Verification items for the finished model (mm, model axes). A direction names the side the tool comes from. Round coordinates to 2 decimals unless told otherwise and drop trailing zeros. Write each loop counter-clockwise with the first axis right and the second up, starting at its lowest first coordinate (ties: lowest second). Pieces come first, ordered by that corner, then holes. Notation, with made-up numbers: (52, -5.75) - (100, -5.75) arc R16 cw to (100, 19.25) - close; hole circle Ø7 at (89.25, 61.5). An arc over 180 degrees is marked (long way). Answer as a JSON object with one key per item and string values.
```python
from build123d import *

# Parameters (mm, degrees)
SKETCH_1_R          = 12.25
SKETCH_1_R_2        = 1.25
EXTRUDE_1_DEPTH     = 2
SKETCH_2_R          = 3
EXTRUDE_2_DEPTH     = 10.63
SKETCH_3_W          = 2
SKETCH_3_H          = 12
EXTRUDE_3_DEPTH     = 8
SKETCH_5_R          = 1.6
CUT_EXTRUDE_1_DEPTH = 10
SKETCH_6_W          = 6
SKETCH_6_H          = 12
EXTRUDE_4_DEPTH     = 10.63
SKETCH_7_W          = 4
SKETCH_7_H          = 12
CUT_EXTRUDE_2_DEPTH = 2


with BuildPart() as part:
    # 草图1 → 凸台-拉伸1 (new body)
    with BuildSketch(Plane(origin=(0, 0, 0), x_dir=(1, 0, 0), z_dir=(0, 1, 0))):
        Circle(SKETCH_1_R)
        with Locations((8, 0)):
            Circle(SKETCH_1_R_2, mode=Mode.SUBTRACT)
        with Locations((0, -8)):
            Circle(SKETCH_1_R_2, mode=Mode.SUBTRACT)
        with Locations((-8, 0)):
            Circle(SKETCH_1_R_2, mode=Mode.SUBTRACT)
        with Locations((0, 8)):
            Circle(SKETCH_1_R_2, mode=Mode.SUBTRACT)
    extrude(amount=EXTRUDE_1_DEPTH)

    # 草图2 → 凸台-拉伸2 (add)
    with BuildSketch(Plane(origin=(0, 2, 0), x_dir=(1, 0, 0), z_dir=(0, 1, 0))):
        Circle(SKETCH_2_R)
    extrude(amount=EXTRUDE_2_DEPTH)

    # 草图3 → 凸台-拉伸3 (add)
    with BuildSketch(Plane(origin=(0, 12.63, 0), x_dir=(1, 0, 0), z_dir=(0, 1, 0))):
        with Locations((-2, 0)):
            Rectangle(SKETCH_3_W, SKETCH_3_H)
    extrude(amount=EXTRUDE_3_DEPTH)

    # 草图5 → 切除-拉伸1 (cut)
    with BuildSketch(Plane(origin=(-1, 0, 0), x_dir=(0, 0, -1), z_dir=(1, 0, 0))):
        with Locations((3, 16.63)):
            Circle(SKETCH_5_R)
        with Locations((-3, 16.63)):
            Circle(SKETCH_5_R)
    extrude(amount=-CUT_EXTRUDE_1_DEPTH, mode=Mode.SUBTRACT)

    # 草图6 → 凸台-拉伸4 (add)
    with BuildSketch(Plane(origin=(0, 2, 0), x_dir=(1, 0, 0), z_dir=(0, 1, 0))):
        Rectangle(SKETCH_6_W, SKETCH_6_H)
    extrude(amount=EXTRUDE_4_DEPTH)

    # 草图7 → 切除-拉伸2 (cut)
    with BuildSketch(Plane(origin=(0, 12.63, 0), x_dir=(1, 0, 0), z_dir=(0, 1, 0))):
        with Locations((1, 0)):
            Rectangle(SKETCH_7_W, SKETCH_7_H)
    extrude(amount=-CUT_EXTRUDE_2_DEPTH, mode=Mode.SUBTRACT)


solid = part.part
```
Q1. Section check B-B, the plane x = 0. Record the cut outline in (y, z), then the cut area to 3 significant figures.
Geometry check:
{"outline": "(0, -12.25) - (2, -12.25) - (2, -9.25) - (0, -9.25) - close; (0, -6.75) - (2, -6.75) - (2, -6) - (10.63, -6) - (10.63, 6) - (2, 6) - (2, 6.75) - (0, 6.75) - close; (0, 9.25) - (2, 9.25) - (2, 12.25) - (0, 12.25) - close", "area": "143 mm2"}
Q2. Gauge pin test, flat ends, axial feed: P1, Ø4.5, axis at x = 1, z = -2, coming from the +Y side; P2, Ø8, axis at y = 13.5, z = -2.5, coming from the +X side; P3, Ø2, axis at x = -8, z = 0, coming from the -Y side; P4, Ø6, axis at x = -4, y = 12.5, coming from the +Z side. Record the tip position at first contact, or that the pin passes through.
Geometry check:
{"P1": "stops at y = 20.63", "P2": "stops at x = 3", "P3": "passes through", "P4": "stops at z = 6"}
Q3. Set-up check for faces 4 (the flat face through (-1, 9, -6)), 5 (the flat face through (3, 6, 0)), 6 (the flat face through (-1, 9, 6)): record each of +Z, -Z, +X, -X, +Y, -Y from which the full face is reachable in a straight line by a thin tool's end or side.
Geometry check:
{"face 4": "-Z, +X, -X, +Y", "face 5": "+Z, -Z, +X, +Y", "face 6": "+Z, +X, -X, +Y"}
Q4. Material ranges on line 1 along Y through (x, z) = (-2.15, 3); line 2 along Z through (x, y) = (0, 0.6); line 3 along X through (y, z) = (6.5, 2.25), recorded low to high. Write a range as [from, to].
Geometry check:
{"line 1": "y = [0, 15.03], [18.23, 20.63]", "line 2": "z = [-12.25, -9.25], [-6.75, 6.75], [9.25, 12.25]", "line 3": "x = [-3, 3]"}
Q5. Release check for a two-part mould opening along Y. For faces 1 (the cylindrical face through (-1.986, 18.216, 3.208)), 2 (the flat face through (-3, 11, 0)), 3 (the flat face through (-2, 20.63, 0)) record: released by +Y, released by -Y, zero draft, split by the parting line, or undercut.
Geometry check:
{"face 1": "undercut", "face 2": "zero draft", "face 3": "released by +Y"}
Q6. Section check D-D, the plane x = 8. Record the cut outline in (y, z).
Geometry check:
{"outline": "(0, -9.28) - (2, -9.28) - (2, -1.25) - (0, -1.25) - close; (0, 1.25) - (2, 1.25) - (2, 9.28) - (0, 9.28) - close"}
Q7. Section check C-C, the plane z = 8. Record the cut outline in (x, y), then the cut area to 3 significant figures.
Geometry check:
{"outline": "(-9.28, 0) - (-1.25, 0) - (-1.25, 2) - (-9.28, 2) - close; (1.25, 0) - (9.28, 0) - (9.28, 2) - (1.25, 2) - close", "area": "32.1 mm2"}
Q8. Section check A-A, the plane y = 16.63. Record the cut outline in (x, z).
Geometry check:
{"outline": "(-3, -6) - (-1, -6) - (-1, -4.6) - (-3, -4.6) - close; (-3, -1.4) - (-1, -1.4) - (-1, 1.4) - (-3, 1.4) - close; (-3, 4.6) - (-1, 4.6) - (-1, 6) - (-3, 6) - close"}
